Build history of the part. All positions in model axes, mm. Give positions to 0.01 mm unless a question says otherwise; leave off trailing zeros. Order: outer loops, then holes, each group sorted by start corner. A loop starts at its lowest first (then second) coordinate and runs counter-clockwise, first axis right, second up. Notation, with made-up numbers: (66.5, 18) - (113.5, 18) arc R15 cw to (113.5, 38) - close; hole circle Ø4 at (66, 87). An arc over 180 degrees is marked (long way). Use a Markdown table: item, result.
from build123d import *

# Parameters (mm, degrees)
F1_DEPTH = 50.8
F2_SIZE  = 49.34077


with BuildPart() as f1:
    # F0 (on Top) → F1 (new body)
    with BuildSketch(Plane.XY):
        Polygon((49.3408840265, 0), (49.3408840265, 28.4869726747), (0, 56.9739453495), (-49.3408840265, 28.4869726747), (-49.3408840265, 0), align=None)
        Polygon((49.3408840265, -28.4869726747), (49.3408840265, 0), (-49.3408840265, 0), (-49.3408840265, -28.4869726747), (0, -56.9739453495), align=None)
    extrude(amount=F1_DEPTH)

    # F2
    f2_edges = [f1.edges().sort_by_distance(p)[0] for p in [
        (24.670442, -42.730459, 50.8),
        (49.340884, 0, 50.8),
        (24.670442, 42.730459, 50.8),
        (-24.670442, 42.730459, 50.8),
        (-49.340884, 0, 50.8),
        (-24.670442, -42.730459, 50.8),
    ]]
    chamfer(f2_edges, length=F2_SIZE)


solid = f1.part
1) Wall check: line 1 (Y direction, x = -11.5, z = 3); line 2 (Y direction, x = 35.5, z = 14.5); line 3 (X direction, y = 22.5, z = 8.5). Give the ranges that are in metal, low to high. Write a range as from..to.
Computed:
| item | result |
|---|---|
| line 1 | y = -48.56..48.56 |
| line 2 | y = -21.42..21.42 |
| line 3 | x = -42.3..42.3 |
2) Slice it at D-D (y = -3.5). Write the cut outline in (x, z), and give its area (3 significant figures).
Computed:
| item | result |
|---|---|
| outline | (-49.34, 0) - (49.34, 0) - (49.34, 1.46) - (6.06, 44.74) - (0, 47.77) - (-6.06, 44.74) - (-49.34, 1.46) - close |
| area | 2,560 mm² |
3) Pin check, flat tips, straight feed: P1, Ø1, axis at x = -10, y = -14, coming from the +Z side; P2, Ø2, axis at x = -22.5, z = 15.5, coming from the -Y side; P3, Ø1.5, axis at x = 19.5, y = 43.5, coming from the -Z side; P4, Ø4, axis at y = 9, z = 36, coming from the -X side. Stop position of each tip, or through.
Computed:
| item | result |
|---|---|
| P1 | stops at z = 34.18 |
| P2 | stops at y = -29.06 |
| P3 | stops at z = 0 |
| P4 | stops at x = -16.8 |
4) Slice it at A-A (y = -17). Write the cut outline in (x, z).
Computed:
| item | result |
|---|---|
| outline | (-49.34, 0) - (49.34, 0) - (49.34, 1.46) - (29.44, 21.36) - (0, 36.08) - (-29.44, 21.36) - (-49.34, 1.46) - close |
5) Slice it at C-C (x = -14.5). Write the cut outline in (y, z), and give its area (3 significant figures).
Computed:
| item | result |
|---|---|
| outline | (-48.6, 0) - (48.6, 0) - (48.6, 1.46) - (8.37, 36.3) - (-8.37, 36.3) - (-48.6, 1.46) - close |
| area | 2,130 mm² |
6) Slice it at B-B (z = 9.5). Write the cut outline in (x, y).
Computed:
| item | result |
|---|---|
| outline | (-41.3, -23.84) - (0, -47.69) - (41.3, -23.84) - (41.3, 23.84) - (0, 47.69) - (-41.3, 23.84) - close |
